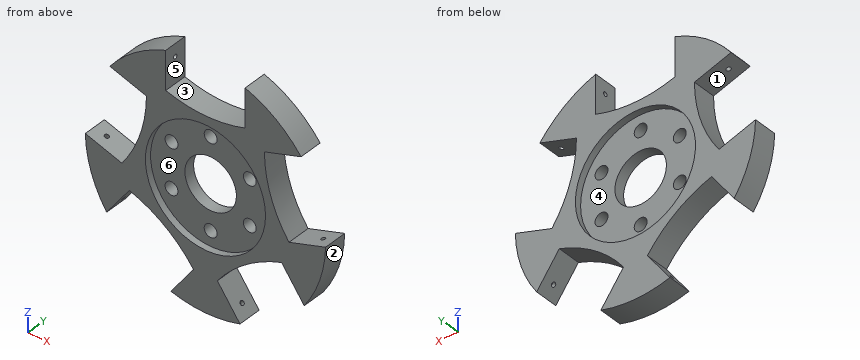
Solid Edge part; units mm, degrees
sketch "Sketch1" plane through (0, 0, 0) normal (0, -1, 0) x (1, 0, 0)
  circle A0 centre (0, 0) radius 28
extrude "Protrusion1" add sketch "Sketch1" along normal mid plane 5.5
sketch "Sketch2" plane through (0, -2.75, 0) normal (0, -1, 0) x (1, 0, 0)
  circle A0 centre (0, 0) radius 14
extrude "Extrusionsausschnitt_1" cut sketch "Sketch2" against normal blind 1.5 and the other way blind 1.5
mirror "Mirror1" about plane through (0, 0, 0) normal (0, -1, 0) of "Extrusionsausschnitt_1"
hole "Bohrung_1" at (-9.1166, -1.25, 5.2095) direction (0, 1, 0) diameter 3 end up to next
hole "Hole1" at (0, -1.25, 10.5) direction (0, 1, 0) diameter 3 end up to next
hole "Hole2" at (9.1225, -1.25, 5.199) direction (0, 1, 0) diameter 3 end up to next
hole "Hole3" at (9.1225, -1.25, -5.199) direction (0, 1, 0) diameter 3 end up to next
hole "Hole4" at (0, -1.25, -10.5) direction (0, 1, 0) diameter 3 end up to next
hole "Hole5" at (-9.1225, -1.25, -5.199) direction (0, 1, 0) diameter 3 end up to next
sketch "Sketch3" plane through (0, -2.75, 0) normal (0, -1, 0) x (1, 0, 0)
  line L0 (-9.25, 23.5) -> (-9.25, 17.46)
  arc A0 (-9.25, 17.46) -> (9.25, 17.46) centre (0, 46.0322) ccw
  line L1 (9.25, 23.5) -> (9.25, 17.46)
  line L2 (9.25, 23.5) -> (9.25, 28.54)
  arc A1 (-9.25, 28.54) -> (9.25, 28.54) centre (0, -0.0322) cw
  line L3 (-9.25, 23.5) -> (-9.25, 28.54)
extrude "Extrusionsausschnitt_3" cut sketch "Sketch3" along normal mid plane 52.8693
pattern_circular "Muster_1" count 5 over 360 about axis through (0, -2.75, 0) along (0, 1, 0) of "Extrusionsausschnitt_3"
sketch "Sketch4" plane through (-9.25, 0, 21.944) normal (1, 0, 0) x (0, 1, 0)
  circle A0 centre (0, 1.556) radius 0.5
extrude "Extrusionsausschnitt_8" cut sketch "Sketch4" against normal blind 1 and the other way blind 1
mirror "Mirror2" about plane through (0, 0, 0) normal (1, 0, 0) of "Extrusionsausschnitt_8"
pattern_circular "Pattern1" count 5 over 360 about axis through (0, -2.75, 0) along (0, 1, 0) of "Extrusionsausschnitt_8", "Mirror2"
hole "Bohrung_7" at (0, -1.25, 0) direction (0, 1, 0) diameter 12 end up to next
properties material "Wheel2"
Could you check a few things on this model? Use its own coordinates, in mm. Face numbers are marked on the shaded views. A direction names the side the tool comes from. Round coordinates to 2 decimals unless told otherwise and drop trailing zeros. Loops run counter-clockwise (first coordinate to the right, second up) from the corner with the lowest first, then second, coordinate; pieces in that order, holes last. Notation, with made-up numbers: (62, 54) -> (114, 54) arc R17 cw to (114, 65) -> close; hole circle Ø5 at (6.5, 78). An arc over 180 degrees is marked (long way). One line per question, with ' | ' between items.
(1) If we section it at B-B on y = 2: List the corners of the cut face in (x, z) for me.
Model answer:
outline: (-27.99, -0.63) arc R28 ccw to (-23.02, -15.94) -> (-17.75, -8.69) arc R30.03 cw to (-2.78, -19.56) -> (-8.05, -26.82) arc R28 ccw to (8.05, -26.82) -> (2.78, -19.56) arc R30.03 cw to (17.75, -8.69) -> (23.02, -15.94) arc R28 ccw to (27.99, -0.63) -> (19.46, -3.4) arc R30.03 cw to (13.75, 14.19) -> (22.28, 16.96) arc R28 ccw to (9.25, 26.43) -> (9.25, 17.46) arc R30.03 cw to (-9.25, 17.46) -> (-9.25, 26.43) arc R28 ccw to (-22.28, 16.96) -> (-13.75, 14.19) arc R30.03 cw to (-19.46, -3.4) -> close; hole circle Ø28 at (0, 0)
(2) For pin 1 Ø1.8 at (x, z) = (0, -10.5) entering from +Y; pin 2 Ø2 at (y, z) = (-1, 7.5) entering from -X; pin 3 Ø1.1 at (y, z) = (0, 23.5) entering from +X; pin 4 Ø2 at (y, z) = (1.5, 12.5) entering from -X, each with a flat end and sliding along its axis, tell me the tip position at first contact or that it passes through.
Model answer:
pin 1: passes through | pin 2: stops at x = -14.76 | pin 3: stops at x = 16.04 | pin 4: stops at x = -13.87
(3) Thinking about a two-plate mould opening in X: for the marked faces 1, 2 and 3, which applies, released by +X, released by -X, zero draft, split by the parting line, or undercut?
Model answer:
face 1: released by -X | face 2: released by +X | face 3: undercut
(4) If we section it at A-A on z = 0: List the corners of the cut face in (x, y) for me, and give its area (3 significant figures).
Model answer:
outline: (-17.33, -2.75) -> (-14, -2.75) -> (-14, -1.25) -> (-6, -1.25) -> (-6, 1.25) -> (-14, 1.25) -> (-14, 2.75) -> (-17.33, 2.75) -> close; (6, -1.25) -> (14, -1.25) -> (14, -2.75) -> (17.33, -2.75) -> (17.33, 2.75) -> (14, 2.75) -> (14, 1.25) -> (6, 1.25) -> close | area: 76.6 mm^2
(5) If I drill on probe 1 along Z at (x, y) = (0, 0.25); probe 2 along Z at (x, y) = (10.05, 0); probe 3 along X at (y, z) = (0.2, -14), over which ranges is the centre line in solid material (lowest first)?
Model answer:
probe 1: z = -28 to -12, -9 to -6, 6 to 9, 12 to 16 | probe 2: z = -12.49 to -6.38, -4.02 to 4.02, 6.38 to 23, 24 to 26.13 | probe 3: x = -24.25 to -21.61, -8.04 to 8.04, 21.61 to 24.25
(6) If we section it at C-C on x = -12.5: List the corners of the cut face in (y, z) for me, and give its area (3 significant figures).
Model answer:
outline: (-2.75, -10.97) -> (2.75, -10.97) -> (2.75, -6.3) -> (1.25, -6.3) -> (1.25, 6.3) -> (2.75, 6.3) -> (2.75, 25.05) -> (-2.75, 25.05) -> (-2.75, 6.3) -> (-1.25, 6.3) -> (-1.25, -6.3) -> (-2.75, -6.3) -> close | area: 160 mm^2
(7) If we section it at D-D on z = 18.5: List the corners of the cut face in (x, y) for me.
Model answer:
outline: (-21.02, -2.75) -> (-9.25, -2.75) -> (-9.25, 2.75) -> (-21.02, 2.75) -> close; (9.25, -2.75) -> (21.02, -2.75) -> (21.02, 2.75) -> (9.25, 2.75) -> close
(8) For the marked faces 4, 5 and 6, which set-ups out of +Z, -Z, +X, -X, +Y, -Y let a thin tool reach every point of the face, with its end or its side?
Model answer:
face 4: +Y | face 5: +Z, +Y, -Y | face 6: -Y
